```python
from build123d import *

# Parameters (mm, degrees)
SKETCH1_W           = 50
SKETCH1_H           = 25
BOSS_EXTRUDE1_DEPTH = 3
SKETCH2_W           = 4.1
SKETCH2_H           = 19.8
BOSS_EXTRUDE2_DEPTH = 12
CHAMFER3_SIZE       = 1
CHAMFER1_SIZE       = 2
FILLET1_R           = 1
SKETCH3_W           = 7.45
SKETCH3_H           = 9.55
CUT_EXTRUDE1_DEPTH  = 38.743078836
CHAMFER2_SIZE       = 1


with BuildPart() as part:
    # Sketch1 → Boss-Extrude1 (new body)
    with BuildSketch(Plane(origin=(0, 0, 0), x_dir=(1, 0, 0), z_dir=(0, 1, 0))):
        Rectangle(SKETCH1_W, SKETCH1_H)
    extrude(amount=BOSS_EXTRUDE1_DEPTH)

    # Sketch2 → Boss-Extrude2 (add)
    with BuildSketch(Plane(origin=(0, 3, 0), x_dir=(1, 0, 0), z_dir=(0, 1, 0))):
        with Locations((-5.25, 0)):
            Rectangle(SKETCH2_W, SKETCH2_H)
        with Locations((5.25, 0)):
            Rectangle(SKETCH2_W, SKETCH2_H)
    extrude(amount=BOSS_EXTRUDE2_DEPTH)

    # Chamfer3
    chamfer3_edges = [part.edges().sort_by_distance(p)[0] for p in [
        (25, 1.5, 12.5),
        (-25, 1.5, 12.5),
        (-25, 1.5, -12.5),
        (25, 1.5, -12.5),
    ]]
    chamfer(chamfer3_edges, length=CHAMFER3_SIZE)

    # Chamfer1
    # the kernel refuses this chamfer: 2 mm, written as the material it takes off along each edge
    with BuildSketch(Plane(origin=(-29.143365976, 0, -12.5), x_dir=(0, 0.9996219169112968, -0.027495876610586494), z_dir=(1, 0, 0))) as chamfer1_piece_1:
        Polygon((CHAMFER1_SIZE * 0.999621916911, CHAMFER1_SIZE * 0.0274958766106), (-CHAMFER1_SIZE * 0.0274958766106, CHAMFER1_SIZE * 0.999621916911), (0, 0), align=None)
    extrude(amount=58.286731952, mode=Mode.SUBTRACT)
    with BuildSketch(Plane(origin=(-25, 0, 16.643365976), x_dir=(0.9996219169112968, -0.02749587661058639, 0), z_dir=(0, 0, -1)), Plane(origin=(25, 0, -16.643365976), x_dir=(-0.9996219169112968, -0.02749587661058639, 0), z_dir=(0, 0, 1))) as chamfer1_piece_2:
        Polygon((CHAMFER1_SIZE * 0.999621916911, -CHAMFER1_SIZE * 0.0274958766106), (-CHAMFER1_SIZE * 0.0274958766106, -CHAMFER1_SIZE * 0.999621916911), (0, 0), align=None)
    extrude(amount=33.286731952, mode=Mode.SUBTRACT)
    with BuildSketch(Plane(origin=(29.143365976, 0, 12.5), x_dir=(0, -0.027495876610586365, -0.9996219169112968), z_dir=(-1, 0, 0))) as chamfer1_piece_3:
        Polygon((CHAMFER1_SIZE * 0.999621916911, -CHAMFER1_SIZE * 0.0274958766106), (-CHAMFER1_SIZE * 0.0274958766106, -CHAMFER1_SIZE * 0.999621916911), (0, 0), align=None)
    extrude(amount=58.286731952, mode=Mode.SUBTRACT)

    # Fillet1
    fillet1_edges = [part.edges().sort_by_distance(p)[0] for p in [
        (0, 2, -12.5),
        (-24.75, 1.75, -11.75),
        (-24.25, 1.75, -12.25),
        (23, 0, 0),
        (0, 0, 10.5),
        (-23, 0, 0),
        (0, 0, -10.5),
        (24.75, 1.75, -11.75),
        (24.25, 1.75, -12.25),
        (-25, 2, 0),
        (-24.25, 1.75, 12.25),
        (-24.75, 1.75, 11.75),
        (0, 2, 12.5),
        (24.75, 1.75, 11.75),
        (24.25, 1.75, 12.25),
        (25, 2, 0),
        (23.75, 0.75, 11.25),
        (-23.75, 0.75, 11.25),
        (23.75, 0.75, -11.25),
        (-23.75, 0.75, -11.25),
    ]]
    fillet(fillet1_edges, radius=FILLET1_R)

    # Sketch3 → Cut-Extrude1 (cut, through all)
    with BuildSketch(Plane.ZY.offset(7.3)):
        with Locations((-3.725, 10.225)):
            Rectangle(SKETCH3_W, SKETCH3_H)
        with Locations((3.725, 10.225)):
            Rectangle(SKETCH3_W, SKETCH3_H)
    extrude(amount=-CUT_EXTRUDE1_DEPTH, mode=Mode.SUBTRACT)

    # Chamfer2
    chamfer2_edges = [part.edges().sort_by_distance(p)[0] for p in [
        (-7.3, 9, -9.9),
        (-7.3, 9, 9.9),
        (7.3, 9, 9.9),
        (7.3, 9, -9.9),
    ]]
    chamfer(chamfer2_edges, length=CHAMFER2_SIZE)


solid = part.part
```
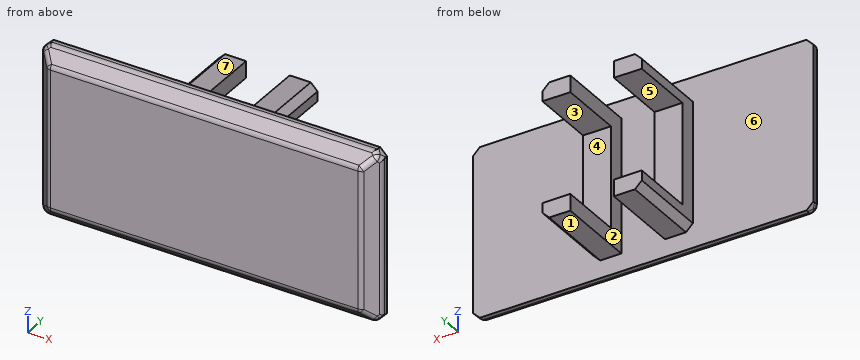
Can you work these out from the model? Positions are in its coordinate system, mm. Face numbers are marked on the shaded views. A direction names the side the tool comes from. Coordinates: 2 decimals unless noted, no trailing zeros. Loops run counter-clockwise (first coordinate to the right, second up) from the corner with the lowest first, then second, coordinate; pieces in that order, holes last. Notation, with made-up numbers: M 21.25,0.5 L 28.25,0.5 A18 cw 28.25,24.5 Z; hole C 75.25,88 d6. An arc over 180 degrees is marked long. Put each result on its own line as item: value. Start each with the question number.
(1) Which directions (+Z, -Z, +X, -X, +Y, -Y) give clear straight access to the entire face, cutting with the end or side of a thin tool? Please do the marked faces 1, 2 and 3.
(2) Will these pins go through, and if not, where does the flat tip stop? pin 1 Ø3.5 at (x, y) = (5.5, 12.5) entering from +Z; pin 2 Ø1 at (x, z) = (19, 4) entering from +Y; pin 3 Ø1.5 at (x, y) = (-4.5, 9.5) entering from -Z.
(3) Imagine slicing it at A-A on y = 6. List the corners of the cut face in (x, z) for me, and give its area (3 significant figures).
(4) Imagine slicing it at B-B on z = 5. List the corners of the cut face in (x, y) for me, and give its area (3 significant figures).
(5) Imagine slicing it at C-C on x = -19. List the corners of the cut face in (y, z) for me.
(6) I need wall thicknesses on probe 1 along Z at (x, y) = (-4, 6.75); probe 2 along X at (y, z) = (8, -8.75); probe 3 along Y at (x, z) = (19.5, -9). Which ranges of each line are inside material? Lowest first, please.
(7) Imagine slicing it at D-D on z = -8. List the corners of the cut face in (x, y) for me.
(8) We'd pull the mould along Z, two halves only. Please class the marked faces 4, 5, 6 and 7: +Z half, -Z half, draft (parallel to the pull), parting line (faces both ways), or undercut.
Worked answers:
1. face 1: -Z, +X, -X, +Y
1. face 2: +Z, -Z, +Y
1. face 3: +X, -X, +Y
2. pin 1: stops at z = 9.9
2. pin 2: stops at y = 3
2. pin 3: stops at z = -9.9
3. outline: M -7.3,-8.9 L -6.3,-9.9 L -3.2,-9.9 L -3.2,-7.45 L -7.3,-7.45 Z; M -7.3,7.45 L -3.2,7.45 L -3.2,9.9 L -6.3,9.9 L -7.3,8.9 Z; M 3.2,-9.9 L 6.3,-9.9 L 7.3,-8.9 L 7.3,-7.45 L 3.2,-7.45 Z; M 3.2,7.45 L 7.3,7.45 L 7.3,8.9 L 6.3,9.9 L 3.2,9.9 Z
3. area: 38.2 mm2
4. outline: M -25,2.41 A1 ccw -24.71,1.71 L -23.29,0.29 A1 ccw -22.59,0 L 22.59,0 A1 ccw 23.29,0.29 L 24.71,1.71 A1 ccw 25,2.41 L 25,3 L 7.3,3 L 7.3,5.45 L 3.2,5.45 L 3.2,3 L -3.2,3 L -3.2,5.45 L -7.3,5.45 L -7.3,3 L -25,3 Z
4. area: 166 mm2
5. outline: M 0,-10.09 A1 ccw 0.29,-10.79 L 1.71,-12.21 A1 ccw 2.41,-12.5 L 3,-12.5 L 3,12.5 L 2.41,12.5 A1 ccw 1.71,12.21 L 0.29,10.79 A1 ccw 0,10.09 Z
6. probe 1: z = -9.9 to -7.45, 7.45 to 9.9
6. probe 2: x = -7.3 to -3.2, 3.2 to 7.3
6. probe 3: y = 0 to 3
7. outline: M -25,2.41 A1 ccw -24.71,1.71 L -23.29,0.29 A1 ccw -22.59,0 L 22.59,0 A1 ccw 23.29,0.29 L 24.71,1.71 A1 ccw 25,2.41 L 25,3 L 7.3,3 L 7.3,15 L 3.2,15 L 3.2,3 L -3.2,3 L -3.2,15 L -7.3,15 L -7.3,3 L -25,3 Z
8. face 4: undercut
8. face 5: undercut
8. face 6: draft
8. face 7: +Z half
